```python
from build123d import *

# Parameters (mm, degrees)
F0_R        = 25.4
F0_R_2      = 21.43125
F0_R_3      = 18.25625
F1_DEPTH    = 66.675
F2_DEPTH    = 84.1375
F3_R        = 6.35
F4_S5_R     = 18.25625
F4_T6_DEPTH = 38
F5_START    = 71.4375
F5_DEPTH    = 12.7


# Not quite as in the source:
# - a fillet or chamfer that OpenCascade refuses, or shapes differently, is made with other operations: its cross-section is extruded or revolved along the edge and cut away or added


with BuildPart() as f1:
    # F0 (on Top) → F1 (new body)
    with BuildSketch(Plane.XY):
        Circle(F0_R)
        Circle(F0_R_2, mode=Mode.SUBTRACT)
        Circle(F0_R_2)
        Circle(F0_R_3, mode=Mode.SUBTRACT)
    extrude(amount=F1_DEPTH)

    # F0 (on Top) → F2 (join)
    with BuildSketch(Plane.XY):
        Circle(F0_R_3)
    extrude(amount=F2_DEPTH)

    # F3
    f3_edges = [f1.edges().sort_by_distance(p)[0] for p in [
        (-25.4, 0, 0),
    ]]
    fillet(f3_edges, radius=F3_R)

    # F4: chamfer of 7.9375 x 15.875 on 1 edges, made by hand


with BuildPart() as f4_tool2:
    # F4_s3 → F4_t4 (revolve)
    with BuildSketch(Plane.XZ):
        Polygon((25.4, 50.8), (17.4625, 66.675), (25.4, 66.675), align=None)
    revolve(axis=Axis((0, 0, 66.675), (0, 0, 1)))

    # F4_s5 → F4_t6 (cut, symmetric)
    with BuildSketch(Plane.XY.offset(58.7)):
        Circle(F4_S5_R)
    extrude(amount=F4_T6_DEPTH, both=True, mode=Mode.SUBTRACT)


with BuildPart() as f1_1:
    add(f1.part)

    # F4_t1: cut F4_tool2
    add(f4_tool2.part, mode=Mode.SUBTRACT)

    # F0 (on Top) → F5 (join)
    with BuildSketch(Plane.XY.offset(F5_START)):
        Circle(F0_R_2)
        Circle(F0_R_3, mode=Mode.SUBTRACT)
    extrude(amount=F5_DEPTH)


solid = f1_1.part
```
Source: CAD feature listing. Evaluate the final solid. Frame: model axes, mm. A direction names the side the tool comes from. Give positions to 0.01 mm unless a question says otherwise; leave off trailing zeros. Write each loop counter-clockwise with the first axis right and the second up, starting at its lowest first coordinate (ties: lowest second). Pieces come first, ordered by that corner, then holes. Notation, with made-up numbers: (-3.75, 77.25) - (13.25, 77.25) arc R5 cw to (13.25, 85.25) - close; hole circle Ø2 at (7.5, 85.25). An arc over 180 degrees is marked (long way). One line per item, written item: value. Start each with the question number.
Q1. Section query A-A, the plane x = 0. Return the cut outline in (y, z).
Q2. Set-up query: faces 4 (the face through (17.744, 5.588, 64.394)), 5 (the face through (0, 0, 84.138)), 6 (the face through (11.52, 18.07, 77.7)). Return all of +Z, -Z, +X, -X, +Y, -Y with unobstructed straight access to the full face (end or side cutting, diameter ignored); none if empty.
Q3. Draft query along Z for faces 1 (the face through (-5.506, -24.796, 28.264)), 2 (the face through (0, 0, 0)), 3 (the face through (16, 10, 71.438)). Return one class per face: +Z half, -Z half, draft (parallel to the pull), parting line (faces both ways), or undercut.
Q4. First-contact query: pin 1 Ø2 at (x, z) = (0.5, 59.5) entering from -Y; pin 2 Ø6 at (x, z) = (2, 20) entering from +Y; pin 3 Ø1.5 at (y, z) = (10, 42.5) entering from +X. Flat tips, straight axial feed; report the tip coordinate or a pass-through.
Q5. Section query D-D, the plane z = 68. Return the cut outline in (x, y).
Q6. Section query C-C, the plane z = 47. Return the cut outline in (x, y).
Q7. Material intervals for probe 1 along X at (y, z) = (-0.5, 12); probe 2 along Z at (x, y) = (-12, -17); probe 3 along Z at (x, y) = (-18.5, 3), sorted ascending. Write a range as from..to.
Answer:
1. outline: (-25.4, 6.35) arc R6.35 ccw to (-19.05, 0) - (19.05, 0) arc R6.35 ccw to (25.4, 6.35) - (25.4, 50.8) - (18.26, 65.09) - (18.26, 71.44) - (21.43, 71.44) - (21.43, 84.14) - (-21.43, 84.14) - (-21.43, 71.44) - (-18.26, 71.44) - (-18.26, 65.09) - (-25.4, 50.8) - close
2. face 4: none
2. face 5: +Z, +X, -X, +Y, -Y
2. face 6: +Z
3. face 1: draft
3. face 2: -Z half
3. face 3: undercut
4. pin 1: stops at y = -21.54
4. pin 2: stops at y = 25.4
4. pin 3: stops at x = 23.66
5. outline: circle Ø36.51 at (0, 0)
6. outline: circle Ø50.8 at (0, 0)
7. probe 1: x = -25.4..25.4
7. probe 2: z = 0.25..59.98, 71.44..84.14
7. probe 3: z = 0..64.12, 71.44..84.14
